from build123d import *

# Parameters (mm, degrees)
ESQUISSE1_W             = 15.8
ESQUISSE1_H             = 8
BOSS_EXTRU_1_DEPTH      = 3.2
ESQUISSE2_R             = 2.4
BOSS_EXTRU_2_DEPTH      = 1.7
ESQUISSE3_R             = 1.9
ENL_V_MAT_EXTRU_1_DEPTH = 1.7
CONG_1_R                = 0.2


with BuildPart() as part:
    # Esquisse1 → Boss.-Extru.1 (new body)
    with BuildSketch(Plane(origin=(0, 0, 0), x_dir=(1, 0, 0), z_dir=(0, 1, 0))):
        with Locations((7.9, 4)):
            Rectangle(ESQUISSE1_W, ESQUISSE1_H)
    extrude(amount=BOSS_EXTRU_1_DEPTH)

    # Esquisse2 → Boss.-Extru.2 (add)
    with BuildSketch(Plane(origin=(0, 3.2, 0), x_dir=(1, 0, 0), z_dir=(0, 1, 0))):
        with Locations(Location((3.95, 4, 0), (0, 0, 90))):
            Circle(ESQUISSE2_R)
        with Locations(Location((11.85, 4, 0), (0, 0, 90))):
            Circle(ESQUISSE2_R)
    extrude(amount=BOSS_EXTRU_2_DEPTH)

    # Esquisse3 → Enlèv. mat.-Extru.1 (cut)
    with BuildSketch(Plane.XZ):
        with Locations(Location((3.95, -4, 0), (0, 0, 270))):
            Circle(ESQUISSE3_R)
        with Locations(Location((11.85, -4, 0), (0, 0, 270))):
            Circle(ESQUISSE3_R)
    extrude(amount=-ENL_V_MAT_EXTRU_1_DEPTH, mode=Mode.SUBTRACT)

    # Congé1
    cong_1_edges = [part.edges().sort_by_distance(p)[0] for p in [
        (3.95, 4.9, -1.6),
        (11.85, 4.9, -1.6),
        (3.95, 1.7, -2.1),
        (11.85, 1.7, -2.1),
    ]]
    fillet(cong_1_edges, radius=CONG_1_R)


solid = part.part
Source: CAD feature listing. Evaluate the final solid. Frame: model axes, mm. A direction names the side the tool comes from. Give positions to 0.01 mm unless a question says otherwise; leave off trailing zeros. Write each loop counter-clockwise with the first axis right and the second up, starting at its lowest first coordinate (ties: lowest second). Pieces come first, ordered by that corner, then holes. Notation, with made-up numbers: (58.25, -32) - (83.25, -32) arc R14 cw to (83.25, -8) - close; hole circle Ø6 at (38, 2). An arc over 180 degrees is marked (long way). Write item = value, one per line. Start each with the question number.
Q1. Cut plane B-B, the plane y = 0.9. Return loops of the section in (x, z).
Q2. Reachability of faces 1 (the cylindrical face through (1.926, 3.94, -5.29)), 2 (the flat face through (8, 2, -8)), 3 (the cylindrical face through (5.234, 0.74, -2.6)) from +Z, -Z, +X, -X, +Y, -Y: full face, straight path, thin tool, end or side. Return the list, or none.
Q3. Draft query along X for faces 4 (the flat face through (12, 1.7, -4)), 5 (the flat face through (8, 3.2, -4)), 6 (the flat face through (15.8, 2, -4)), 7 (the flat face through (8, 2, 0)). Return one class per face: +X half, -X half, draft (parallel to the pull), parting line (faces both ways), or undercut.
Q4. Cut plane D-D, the plane y = 4.2. Return loops of the section in (x, z).
Q5. Pin query (flat end, axial travel): pin 1 Ø1 at (x, z) = (11.5, -4) entering from -Y; pin 2 Ø1.5 at (y, z) = (4, -6.5) entering from -X. Return the tip coordinate at first contact, or that it passes through.
Q6. Cut plane C-C, the plane z = -4. Return loops of the section in (x, y), then the cut area to 3 significant figures.
Q7. Material intervals for probe 1 along X at (y, z) = (0.7, -4); probe 2 along Y at (x, z) = (3, -7); probe 3 along Z at (x, y) = (4, 1.2), sorted ascending.
Q8. Cut plane A-A, the plane x = 11.85. Return loops of the section in (y, z).
Computed values:
q1.outline = (0, -8) - (15.8, -8) - (15.8, 0) - (0, 0) - close; hole circle Ø3.8 at (3.95, -4); hole circle Ø3.8 at (11.85, -4)
q2.face_1 = +Y
q2.face_2 = -Z, +X, -X, +Y, -Y
q2.face_3 = -Y
q3.face_4 = undercut
q3.face_5 = undercut
q3.face_6 = +X half
q3.face_7 = draft
q4.outline = circle Ø4.8 at (3.95, -4); circle Ø4.8 at (11.85, -4)
q5.pin_1 = 1.7
q5.pin_2 = 2.31
q6.outline = (0, 0) - (2.05, 0) - (2.05, 1.5) arc R0.2 cw to (2.25, 1.7) - (5.65, 1.7) arc R0.2 cw to (5.85, 1.5) - (5.85, 0) - (9.95, 0) - (9.95, 1.5) arc R0.2 cw to (10.15, 1.7) - (13.55, 1.7) arc R0.2 cw to (13.75, 1.5) - (13.75, 0) - (15.8, 0) - (15.8, 3.2) - (14.25, 3.2) - (14.25, 4.7) arc R0.2 ccw to (14.05, 4.9) - (9.65, 4.9) arc R0.2 ccw to (9.45, 4.7) - (9.45, 3.2) - (6.35, 3.2) - (6.35, 4.7) arc R0.2 ccw to (6.15, 4.9) - (1.75, 4.9) arc R0.2 ccw to (1.55, 4.7) - (1.55, 3.2) - (0, 3.2) - close
q6.area = 54.0 mm²
q7.probe_1 = 0 to 2.05, 5.85 to 9.95, 13.75 to 15.8
q7.probe_2 = 0 to 3.2
q7.probe_3 = -8 to -5.9, -2.1 to 0
q8.outline = (0, -8) - (3.2, -8) - (3.2, -6.4) - (4.7, -6.4) arc R0.2 ccw to (4.9, -6.2) - (4.9, -1.8) arc R0.2 ccw to (4.7, -1.6) - (3.2, -1.6) - (3.2, 0) - (0, 0) - (0, -2.1) - (1.5, -2.1) arc R0.2 cw to (1.7, -2.3) - (1.7, -5.7) arc R0.2 cw to (1.5, -5.9) - (0, -5.9) - close
